Verification items for the finished model (mm, model axes). A direction names the side the tool comes from. Coordinates: 2 decimals unless noted, no trailing zeros. Order: outer loops, then holes, each group sorted by start corner. A loop starts at its lowest first (then second) coordinate and runs counter-clockwise, first axis right, second up. Notation, with made-up numbers: M 56,-1 L 67,-1 A26 ccw 67,26 Z; hole C 53.5,81 d4. An arc over 180 degrees is marked long. Return JSON: item names as keys, results as strings. Group by question number.
1. Section check A-A, the plane y = 2.8. Record the cut outline in (x, z), plus the area to 3 significant figures.
2. Material ranges on line 1 along X through (y, z) = (2.5, 3); line 2 along Y through (x, z) = (14.5, 4); line 3 along Y through (x, z) = (-6, 4.5), recorded low to high.
3. Mould release check, pull along Y, two halves, no side actions. Record for faces 1 (the flat face through (0, 1, 6.502)), 2 (the flat face through (-13, 3.5, 3)), 3 (the flat face through (0, 0, 3)): +Y half, -Y half, draft (parallel to the pull), parting line (faces both ways), or undercut.
4. Gauge pin test, flat ends, axial feed: pin 1 (1.6 mm diameter, centred on y = 3, z = 3, fed in from +X); pin 2 (0.8 mm diameter, centred on y = 3, z = 2.5, fed in from -X); pin 3 (1.2 mm diameter, centred on x = 8.5, y = 3.5, fed in from -Z). Record the tip position at first contact, or that the pin passes through.
5. Section check D-D, the plane x = -4.5. Record the cut outline in (y, z), plus the area to 3 significant figures.
6. Section check B-B, the plane x = 15.5. Record the cut outline in (y, z), plus the area to 3 significant figures.
7. Set-up check for faces 4 (the flat face through (-6.564, 3, 3)), 5 (the flat face through (18.391, 3, 3)), 6 (the flat face through (11, 4, 4.159)): record each of +Z, -Z, +X, -X, +Y, -Y from which the full face is reachable in a straight line by a thin tool's end or side.
8. Section check C-C, the plane z = 2.75. Record the cut outline in (x, y).
```python
from build123d import *

# Parameters (mm, degrees)
SKETCH1_W           = 47.678483764
SKETCH1_H           = 13.004323218
BOSS_EXTRUDE1_DEPTH = 2
SKETCH2_W           = 1.5
SKETCH2_H           = 2.5
BOSS_EXTRUDE2_DEPTH = 1.5
SKETCH3_W           = 12
SKETCH3_H           = 2.5
SKETCH3_W_2         = 18
BOSS_EXTRUDE3_DEPTH = 1
SKETCH4_W           = 47.678483764
SKETCH4_H           = 6.502161609
CUT_EXTRUDE1_DEPTH  = 25.83621467


with BuildPart() as part:
    # Sketch1 → Boss-Extrude1 (new body)
    with BuildSketch(Plane(origin=(0, 0, 0), x_dir=(1, 0, 0), z_dir=(0, 1, 0))):
        Rectangle(SKETCH1_W, SKETCH1_H)
    extrude(amount=BOSS_EXTRUDE1_DEPTH)

    # Sketch2 → Boss-Extrude2 (add)
    with BuildSketch(Plane(origin=(0, 2, 0), x_dir=(1, 0, 0), z_dir=(0, 1, 0))):
        with Locations((-17.814028346, -2.908609225)):
            Rectangle(SKETCH2_W, SKETCH2_H)
        with Locations((-7.314028346, -2.908609225)):
            Rectangle(SKETCH2_W, SKETCH2_H)
        with Locations((2.641012715, -2.908609225)):
            Rectangle(SKETCH2_W, SKETCH2_H)
        with Locations((19.141012715, -2.908609225)):
            Rectangle(SKETCH2_W, SKETCH2_H)
    extrude(amount=BOSS_EXTRUDE2_DEPTH)

    # Sketch3 → Boss-Extrude3 (add)
    with BuildSketch(Plane(origin=(0, 3.5, 0), x_dir=(1, 0, 0), z_dir=(0, 1, 0))):
        with Locations((-12.564028346, -2.908609225)):
            Rectangle(SKETCH3_W, SKETCH3_H)
        with Locations((10.891012715, -2.908609225)):
            Rectangle(SKETCH3_W_2, SKETCH3_H)
    extrude(amount=BOSS_EXTRUDE3_DEPTH)

    # Sketch4 → Cut-Extrude1 (cut, through all)
    with BuildSketch(Plane(origin=(0, 2, 0), x_dir=(1, 0, 0), z_dir=(0, 1, 0))):
        with Locations((0, 3.251080805)):
            Rectangle(SKETCH4_W, SKETCH4_H)
    extrude(amount=-CUT_EXTRUDE1_DEPTH, mode=Mode.SUBTRACT)


solid = part.part
```
Answers follow:
{
 "1": {"outline": "M -18.56,1.66 L -17.06,1.66 L -17.06,4.16 L -18.56,4.16 Z; M -8.06,1.66 L -6.56,1.66 L -6.56,4.16 L -8.06,4.16 Z; M 1.89,1.66 L 3.39,1.66 L 3.39,4.16 L 1.89,4.16 Z; M 18.39,1.66 L 19.89,1.66 L 19.89,4.16 L 18.39,4.16 Z", "area": "15.0 mm^2"},
 "2": {"line 1": "-18.56 to -17.06, -8.06 to -6.56, 1.89 to 3.39, 18.39 to 19.89", "line 2": "0 to 2, 3.5 to 4.5", "line 3": "0 to 2"},
 "3": {"face 1": "draft", "face 2": "undercut", "face 3": "-Y half"},
 "4": {"pin 1": "x = 19.89", "pin 2": "x = -18.56", "pin 3": "z = 1.66"},
 "5": {"outline": "M 0,0 L 2,0 L 2,6.5 L 0,6.5 Z", "area": "13.0 mm^2"},
 "6": {"outline": "M 0,0 L 2,0 L 2,6.5 L 0,6.5 Z; M 3.5,1.66 L 4.5,1.66 L 4.5,4.16 L 3.5,4.16 Z", "area": "15.5 mm^2"},
 "7": {"face 4": "+Z, -Z, +Y", "face 5": "+Z, -Z", "face 6": "+Z, +X, -X, +Y"},
 "8": {"outline": "M -23.84,0 L 23.84,0 L 23.84,2 L 19.89,2 L 19.89,4.5 L 1.89,4.5 L 1.89,2 L -6.56,2 L -6.56,4.5 L -18.56,4.5 L -18.56,2 L -23.84,2 Z; hole M -17.06,2 L -8.06,2 L -8.06,3.5 L -17.06,3.5 Z; hole M 3.39,2 L 18.39,2 L 18.39,3.5 L 3.39,3.5 Z"}
}
